```python
from build123d import *

# Parameters (mm, degrees)
SKETCH1_W            = 10
SKETCH1_H            = 10
SKETCH1_W_2          = 6
SKETCH1_H_2          = 6
BOSS_EXTRUDE1_DEPTH  = 2.54
BOSS_EXTRUDE4_DEPTH  = 2.54
CUT_EXTRUDE4_DEPTH   = 2.54
BOSS_EXTRUDE6_DEPTH  = 2.54
BOSS_EXTRUDE7_DEPTH  = 2.54
SKETCH8_W            = 16
SKETCH8_H            = 16
SKETCH8_W_2          = 12
SKETCH8_H_2          = 12
CUT_EXTRUDE5_DEPTH   = 0.5
SKETCH9_W            = 8
SKETCH9_H            = 8
BOSS_EXTRUDE8_DEPTH  = 0.5
SKETCH10_W           = 12
SKETCH10_H           = 12
SKETCH10_W_2         = 8
SKETCH10_H_2         = 8
CUT_EXTRUDE6_DEPTH   = 10
SKETCH11_W           = 16
SKETCH11_H           = 16
SKETCH11_W_2         = 8
SKETCH11_H_2         = 8
BOSS_EXTRUDE9_DEPTH  = 2
SKETCH13_W           = 8
SKETCH13_H           = 8
CUT_EXTRUDE7_DEPTH   = 2
SKETCH14_W           = 10
SKETCH14_H           = 10
SKETCH14_W_2         = 6
SKETCH14_H_2         = 6
CUT_EXTRUDE8_DEPTH   = 2
SKETCH16_W           = 14
SKETCH16_H           = 14
SKETCH16_W_2         = 12
SKETCH16_H_2         = 12
CUT_EXTRUDE12_DEPTH  = 10
SKETCH17_W           = 18
SKETCH17_H           = 18
SKETCH17_W_2         = 16
SKETCH17_H_2         = 16
BOSS_EXTRUDE10_DEPTH = 4
SKETCH18_W           = 18
SKETCH18_H           = 18
SKETCH18_W_2         = 16
SKETCH18_H_2         = 16
BOSS_EXTRUDE11_DEPTH = 1
SKETCH19_W           = 10
SKETCH19_H           = 10
SKETCH19_W_2         = 6
SKETCH19_H_2         = 6
BOSS_EXTRUDE12_DEPTH = 150
SKETCH20_W           = 10
SKETCH20_H           = 10
BOSS_EXTRUDE13_DEPTH = 2


with BuildPart() as part:
    # Sketch1 → Boss-Extrude1 (new body)
    with BuildSketch(Plane.XY):
        with Locations((3, 3)):
            Rectangle(SKETCH1_W, SKETCH1_H)
        with Locations((3, 3)):
            Rectangle(SKETCH1_W_2, SKETCH1_H_2, mode=Mode.SUBTRACT)
    extrude(amount=BOSS_EXTRUDE1_DEPTH)

    # Sketch2 → Boss-Extrude4 (add)
    with BuildSketch(Plane(origin=(0, 0, 0), x_dir=(-1, 0, 0), z_dir=(0, 0, -1))):
        Polygon((-8, 8), (-8, -2), (2, -2), (2, -4), (-10, -4), (-10, 8), align=None)
    extrude(amount=-BOSS_EXTRUDE4_DEPTH)

    # Sketch5 → Cut-Extrude4 (cut)
    with BuildSketch(Plane(origin=(0, 0, 0), x_dir=(-1, 0, 0), z_dir=(0, 0, -1))):
        Polygon((-6, 6), (-6, 0), (0, 0), (0, -2), (-8, -2), (-8, 6), align=None)
    extrude(amount=-CUT_EXTRUDE4_DEPTH, mode=Mode.SUBTRACT)

    # Sketch6 → Boss-Extrude6 (add)
    with BuildSketch(Plane(origin=(0, 0, 0), x_dir=(-1, 0, 0), z_dir=(0, 0, -1))):
        Polygon((-10, 8), (-10, -4), (2, -4), (2, -6), (-12, -6), (-12, 8), align=None)
    extrude(amount=-BOSS_EXTRUDE6_DEPTH)

    # Sketch7 → Boss-Extrude7 (add)
    with BuildSketch(Plane(origin=(0, 0, 0), x_dir=(-1, 0, 0), z_dir=(0, 0, -1))):
        Polygon((-12, 8), (2, 8), (2, -6), (4, -6), (4, 10), (-12, 10), align=None)
    extrude(amount=-BOSS_EXTRUDE7_DEPTH)

    # Sketch8 → Cut-Extrude5 (cut)
    with BuildSketch(Plane(origin=(0, 0, 0), x_dir=(-1, 0, 0), z_dir=(0, 0, -1))):
        with Locations((-4, 2)):
            Rectangle(SKETCH8_W, SKETCH8_H)
        with Locations((-4, 2)):
            Rectangle(SKETCH8_W_2, SKETCH8_H_2, mode=Mode.SUBTRACT)
    extrude(amount=-CUT_EXTRUDE5_DEPTH, mode=Mode.SUBTRACT)

    # Sketch10 → Cut-Extrude6 (cut)
    with BuildSketch(Plane(origin=(0, 0, 0), x_dir=(-1, 0, 0), z_dir=(0, 0, -1))):
        with Locations((-4, 2)):
            Rectangle(SKETCH10_W, SKETCH10_H)
        with Locations((-4, 2)):
            Rectangle(SKETCH10_W_2, SKETCH10_H_2, mode=Mode.SUBTRACT)
    extrude(amount=-CUT_EXTRUDE6_DEPTH, mode=Mode.SUBTRACT)

    # Sketch11 → Boss-Extrude9 (add)
    with BuildSketch(Plane.XY.offset(2.54)):
        with Locations((4, 2)):
            Rectangle(SKETCH11_W, SKETCH11_H)
        with Locations((4, 2)):
            Rectangle(SKETCH11_W_2, SKETCH11_H_2, mode=Mode.SUBTRACT)
    extrude(amount=BOSS_EXTRUDE9_DEPTH)

    # Sketch14 → Cut-Extrude8 (cut)
    with BuildSketch(Plane(origin=(0, 0, 2.54), x_dir=(-1, 0, 0), z_dir=(0, 0, -1))):
        with Locations((-4, 2)):
            Rectangle(SKETCH14_W, SKETCH14_H)
        with Locations((-4, 2)):
            Rectangle(SKETCH14_W_2, SKETCH14_H_2, mode=Mode.SUBTRACT)
    extrude(amount=-CUT_EXTRUDE8_DEPTH, mode=Mode.SUBTRACT)

    # Sketch16 → Cut-Extrude12 (cut)
    with BuildSketch(Plane(origin=(0, 0, 2.54), x_dir=(-1, 0, 0), z_dir=(0, 0, -1))):
        with Locations((-4, 2)):
            Rectangle(SKETCH16_W, SKETCH16_H)
        with Locations((-4, 2)):
            Rectangle(SKETCH16_W_2, SKETCH16_H_2, mode=Mode.SUBTRACT)
    extrude(amount=CUT_EXTRUDE12_DEPTH, mode=Mode.SUBTRACT)

    # Sketch17 → Boss-Extrude10 (add)
    with BuildSketch(Plane(origin=(0, 0, 0.5), x_dir=(-1, 0, 0), z_dir=(0, 0, -1))):
        with Locations((-4, 2)):
            Rectangle(SKETCH17_W, SKETCH17_H)
        with Locations((-4, 2)):
            Rectangle(SKETCH17_W_2, SKETCH17_H_2, mode=Mode.SUBTRACT)
    extrude(amount=-BOSS_EXTRUDE10_DEPTH)

    # Sketch18 → Boss-Extrude11 (add)
    with BuildSketch(Plane.XY.offset(4.54)):
        with Locations((4, 2)):
            Rectangle(SKETCH18_W, SKETCH18_H)
        with Locations((4, 2)):
            Rectangle(SKETCH18_W_2, SKETCH18_H_2, mode=Mode.SUBTRACT)
    extrude(amount=-BOSS_EXTRUDE11_DEPTH)

    # Sketch19 → Boss-Extrude12 (add)
    with BuildSketch(Plane.XY.offset(4.54)):
        with Locations((4, 2)):
            Rectangle(SKETCH19_W, SKETCH19_H)
        with Locations((4, 2)):
            Rectangle(SKETCH19_W_2, SKETCH19_H_2, mode=Mode.SUBTRACT)
    extrude(amount=-BOSS_EXTRUDE12_DEPTH)

    # Sketch20 → Boss-Extrude13 (add)
    with BuildSketch(Plane(origin=(0, 0, -145.46), x_dir=(-1, 0, 0), z_dir=(0, 0, -1))):
        with Locations((-4, 2)):
            Rectangle(SKETCH20_W, SKETCH20_H)
    extrude(amount=BOSS_EXTRUDE13_DEPTH)


with BuildPart() as body_2:
    # Sketch9 → Boss-Extrude8 (new body)
    with BuildSketch(Plane(origin=(0, 0, 0), x_dir=(-1, 0, 0), z_dir=(0, 0, -1))):
        with Locations((-4, 2)):
            Rectangle(SKETCH9_W, SKETCH9_H)
    extrude(amount=BOSS_EXTRUDE8_DEPTH)

    # Sketch13 → Cut-Extrude7 (cut)
    with BuildSketch(Plane(origin=(0, 0, -0.5), x_dir=(-1, 0, 0), z_dir=(0, 0, -1))):
        with Locations((-4, 2)):
            Rectangle(SKETCH13_W, SKETCH13_H)
    extrude(amount=-CUT_EXTRUDE7_DEPTH, mode=Mode.SUBTRACT)


solid = part.part
```
The listing builds one solid part. Answer for the finished solid, in the listing's coordinates (mm). A direction names the side the tool comes from. Coordinates: 2 decimals unless noted, no trailing zeros. Write each loop counter-clockwise with the first axis right and the second up, starting at its lowest first coordinate (ties: lowest second). Pieces come first, ordered by that corner, then holes. Notation, with made-up numbers: (76.25, 84) - (111.25, 84) arc R34 ccw to (111.25, 123) - close; hole circle Ø11 at (-25.5, 17.25). An arc over 180 degrees is marked (long way). Return JSON: item names as keys, results as strings. Group by question number.
1. Straight lines are drawn through the part: L1, parallel to X at y = 4, z = -93; L2, parallel to Y at x = 6.25, z = -60.5; L3, parallel to X at y = 6, z = -139. For each, find the intervals that lie inside material, in ascending order.
2. Determine the mould class of faces 1 (the flat face through (-5, 2, 3)), 2 (the flat face through (1, 2, -69)), 3 (the flat face through (4, 2, -147.46)) for opening direction X: released by +X, released by -X, zero draft, split by the parting line, or undercut.
3. Given pin 1 (3 mm diameter, centred on y = 4, z = -122.5, fed in from +X); pin 2 (1 mm diameter, centred on x = 3.5, z = -131, fed in from +Y); pin 3 (3 mm diameter, centred on x = 5.5, z = -93, fed in from -Y), each flat-ended and moving along its own axis, determine where each tip first touches the part or whether it passes through.
4. Which of the six approach directions +Z, -Z, +X, -X, +Y, -Y give full straight-line access (tool end or side, diameter ignored) to faces 4 (the flat face through (4, -1, -69)), 5 (the flat face through (12, 2, 0.5)), 6 (the flat face through (4, 11, 3))?
5. A cutting plane is placed at A-A, the plane z = -137. Determine the outline of the cut face in (x, y).
6. A cutting plane is placed at B-B, the plane x = 2.25. Determine the outline of the cut face in (y, z).
7. A cutting plane is placed at C-C, the plane y = 1.25. Determine the outline of the cut face in (x, z).
Ans:
{
 "1": {"L1": "-1 to 1, 7 to 9", "L2": "-3 to -1, 5 to 7", "L3": "-1 to 9"},
 "2": {"face 1": "released by -X", "face 2": "undercut", "face 3": "zero draft"},
 "3": {"pin 1": "x = 9", "pin 2": "y = 7", "pin 3": "y = -3"},
 "4": {"face 4": "+Z", "face 5": "-Z", "face 6": "+Z, -Z, +X, -X, +Y"},
 "5": {"outline": "(-1, -3) - (9, -3) - (9, 7) - (-1, 7) - close; hole (1, -1) - (7, -1) - (7, 5) - (1, 5) - close"},
 "6": {"outline": "(-7, 0.5) - (-5, 0.5) - (-5, 2.54) - (-3, 2.54) - (-3, -147.46) - (7, -147.46) - (7, 2.54) - (9, 2.54) - (9, 0.5) - (11, 0.5) - (11, 4.54) - (5, 4.54) - (5, -145.46) - (-1, -145.46) - (-1, 4.54) - (-7, 4.54) - close"},
 "7": {"outline": "(-5, 0.5) - (-3, 0.5) - (-3, 2.54) - (-1, 2.54) - (-1, -147.46) - (9, -147.46) - (9, 2.54) - (11, 2.54) - (11, 0.5) - (13, 0.5) - (13, 4.54) - (7, 4.54) - (7, -145.46) - (1, -145.46) - (1, 4.54) - (-5, 4.54) - close"}
}
